Job drawing, mm, ordinate dimensions from the low corner. One solid piece. Coordinates: 2 decimals unless noted, no trailing zeros. Write each loop counter-clockwise with the first axis right and the second up, starting at its lowest first coordinate (ties: lowest second). Pieces come first, ordered by that corner, then holes. Notation, with made-up numbers: (-4.5, -30) -> (-0.5, -30) arc R36 cw to (-0.5, 7) -> close; hole circle Ø4 at (32, -22.75). An arc over 180 degrees is marked (long way). Answer as a JSON object with one key per item and string values. Group by question number.
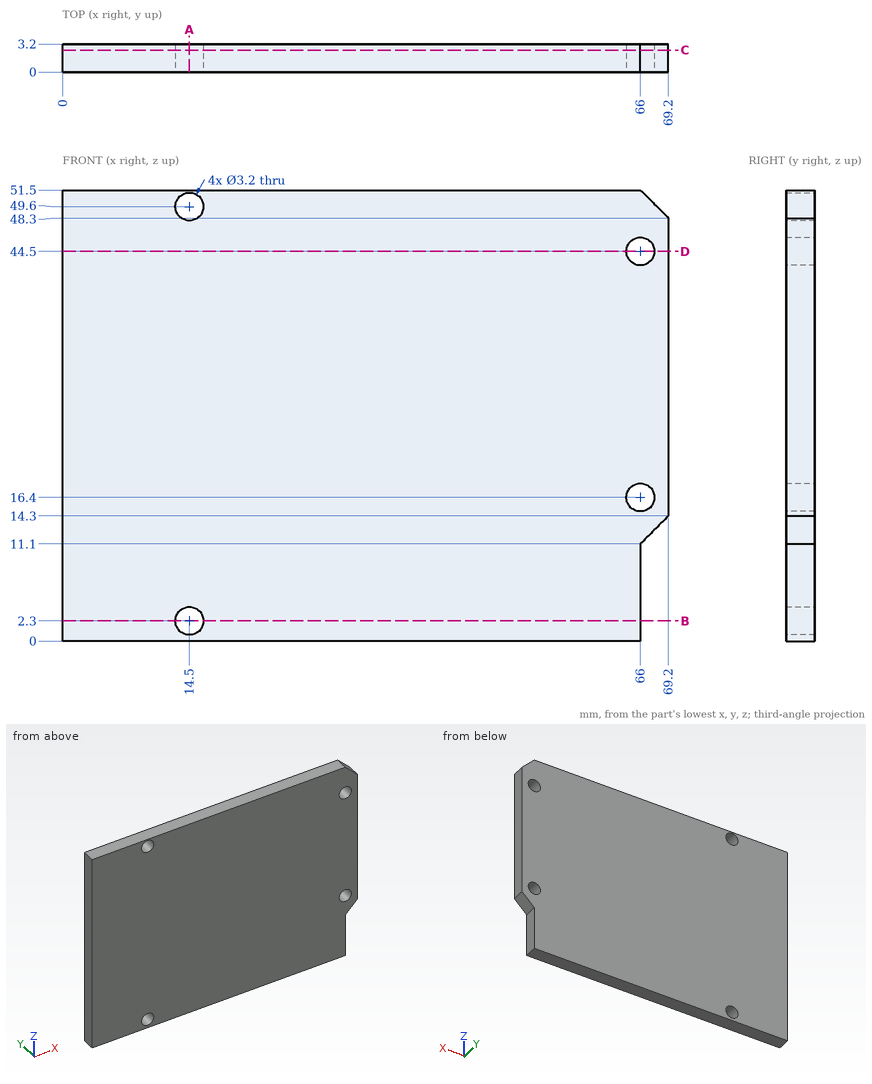
(1) Cut at D-D on z = 44.5. List the corners of the cut face in (x, y), plus the area to 3 significant figures.
(2) Wall check: probe 1 along X at (y, z) = (2.25, 2.3); probe 2 along X at (y, z) = (0.75, 44.5); probe 3 along X at (y, z) = (1.3, 8.5). Give the ranges that are in metal, low to high.
(3) Cut at C-C on y = 2.5. List the corners of the cut face in (x, z).
(4) Pin check, flat tip, straight feed: pin 1 (1 mm diameter, centred on y = 1, z = 5, fed in from +X). Stop position of the tip, or through.
(5) Cut at B-B on z = 2.3. List the corners of the cut face in (x, y), plus the area to 3 significant figures.
(6) Cut at A-A on x = 14.5. List the corners of the cut face in (y, z).
Results found:
{
 "1": {"outline": "(0, 0) -> (64.4, 0) -> (64.4, 3.2) -> (0, 3.2) -> close; (67.6, 0) -> (69.2, 0) -> (69.2, 3.2) -> (67.6, 3.2) -> close", "area": "211 mm²"},
 "2": {"probe 1": "x = 0 to 12.9, 16.1 to 66", "probe 2": "x = 0 to 64.4, 67.6 to 69.2", "probe 3": "x = 0 to 66"},
 "3": {"outline": "(0, 0) -> (66, 0) -> (66, 11.1) -> (69.2, 14.3) -> (69.2, 48.3) -> (66, 51.5) -> (0, 51.5) -> close; hole circle Ø3.2 at (14.5, 2.3); hole circle Ø3.2 at (14.5, 49.6); hole circle Ø3.2 at (66, 16.4); hole circle Ø3.2 at (66, 44.5)"},
 "4": {"pin 1": "stops at x = 66"},
 "5": {"outline": "(0, 0) -> (12.9, 0) -> (12.9, 3.2) -> (0, 3.2) -> close; (16.1, 0) -> (66, 0) -> (66, 3.2) -> (16.1, 3.2) -> close", "area": "201 mm²"},
 "6": {"outline": "(0, 0) -> (3.2, 0) -> (3.2, 0.7) -> (0, 0.7) -> close; (0, 3.9) -> (3.2, 3.9) -> (3.2, 48) -> (0, 48) -> close; (0, 51.2) -> (3.2, 51.2) -> (3.2, 51.5) -> (0, 51.5) -> close"}
}
